Read the model definition and answer for the solid it produces. Units are mm, in the model's axes. Coordinates: 2 decimals unless noted, no trailing zeros. Loops run counter-clockwise (first coordinate to the right, second up) from the corner with the lowest first, then second, coordinate; pieces in that order, holes last. Notation, with made-up numbers: (85, -21) - (119, -21) arc R16 cw to (119, -7) - close; hole circle Ø10 at (-24.75, -12.75). An arc over 180 degrees is marked (long way). Use one line per item in the form item = value. Start each with the question number.
1) A cutting plane is placed at B-B (x = -3.5). Give the vertices of the cut face in (y, z).
2) A cutting plane is placed at A-A (z = 16.5). Give the vertices of the cut face in (x, y), and give its area (3 significant figures).
3) Consider line 1 (Z direction, x = -3.75, y = -0.25); line 2 (Z direction, x = -3.75, y = -2.5); line 3 (Y direction, x = -3, z = 4). Determine where each line is inside the solid, lowest interval first.
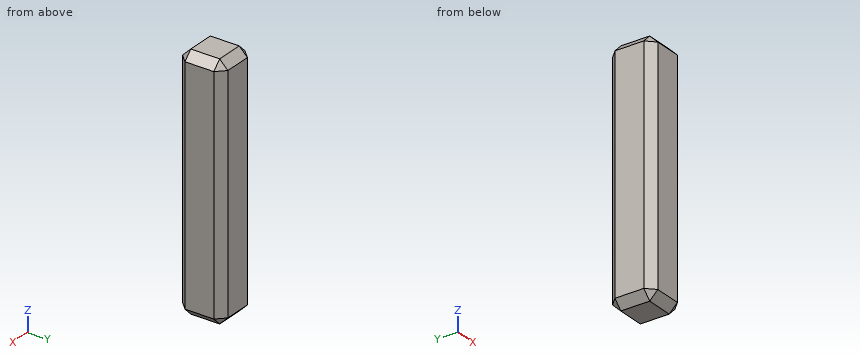
from build123d import *

# Parameters (mm, degrees)
SKETCH1_W           = 8
SKETCH1_H           = 8.3
BOSS_EXTRUDE1_DEPTH = 45
CHAMFER1_SIZE       = 1.5


with BuildPart() as part:
    # Sketch1 → Boss-Extrude1 (new body)
    with BuildSketch(Plane.XY):
        with Locations((-0.340337416, 0.353)):
            Rectangle(SKETCH1_W, SKETCH1_H)
    extrude(amount=BOSS_EXTRUDE1_DEPTH)

    # Chamfer1
    chamfer1_edges = [part.edges().sort_by_distance(p)[0] for p in [
        (3.659662584, 0.353, 45),
        (-0.340337416, 4.503, 45),
        (-4.340337416, 0.353, 45),
        (-0.340337416, 4.503, 0),
        (3.659662584, 0.353, 0),
        (-0.340337416, -3.797, 0),
        (-4.340337416, 0.353, 0),
        (-4.340337416, 4.503, 22.5),
        (3.659662584, 4.503, 22.5),
        (3.659662584, -3.797, 22.5),
        (-4.340337416, -3.797, 22.5),
        (-0.340337416, -3.797, 45),
    ]]
    chamfer(chamfer1_edges, length=CHAMFER1_SIZE)


solid = part.part
Found:
q1.outline = (-3.14, 1.5) - (-2.3, 0.66) - (3, 0.66) - (3.84, 1.5) - (3.84, 43.5) - (3, 44.34) - (-2.3, 44.34) - (-3.14, 43.5) - close
q2.outline = (-4.34, -2.3) - (-2.84, -3.8) - (2.16, -3.8) - (3.66, -2.3) - (3.66, 3) - (2.16, 4.5) - (-2.84, 4.5) - (-4.34, 3) - close
q2.area = 61.9 mm^2
q3.line_1 = 0.91 to 44.09
q3.line_2 = 1.11 to 43.89
q3.line_3 = -3.64 to 4.34
